Here's how the part is built. I have some questions about the finished solid (model axes, mm). Coordinates: 2 decimals unless noted, no trailing zeros. Loops run counter-clockwise (first coordinate to the right, second up) from the corner with the lowest first, then second, coordinate; pieces in that order, holes last. Notation, with made-up numbers: (63, -15.75) - (88, -15.75) arc R19 ccw to (88, 2.25) - close; hole circle Ø3 at (57.25, 16). An arc over 180 degrees is marked (long way). Use a Markdown table: item, result.
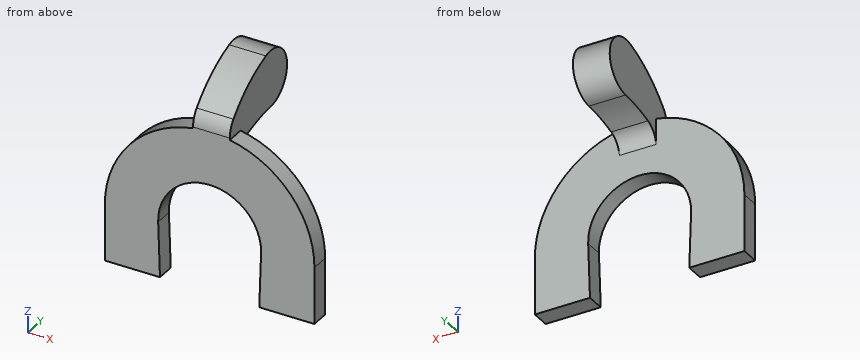
```python
from build123d import *

# Parameters (mm, degrees)
BOSS_EXTRUDE1_DEPTH      = 1
BOSS_EXTRUDE2_START      = 2.8
BOSS_EXTRUDE2_DEPTH      = 1
BOSS_EXTRUDE2_DEPTH_BACK = 1


with BuildPart() as part:
    # Sketch1 → Boss-Extrude1 (new body)
    with BuildSketch(Plane(origin=(0, 0, 0), x_dir=(1, 0, 0), z_dir=(0, 1, 0))):
        with BuildLine():
            Line((0, 0), (-3, 0))
            Line((-3, 0), (-3, -3.090307428))
            ThreePointArc((-3, -3.090307428), (2.7, -8.790307428), (8.4, -3.090307428))
            Line((8.4, -3.090307428), (8.4, 0))
            Line((8.4, 0), (5.4, 0))
            Line((5.4, 0), (5.498490641, -2.99838283))
            ThreePointArc((5.498490641, -2.99838283), (2.7, -5.890307428), (-0.098490641, -2.99838283))
            Line((-0.098490641, -2.99838283), (0, 0))
        make_face()
    extrude(amount=BOSS_EXTRUDE1_DEPTH)

    # Sketch2 → Boss-Extrude2 (add, two sides)
    with BuildSketch(Plane(origin=(0, 0, 0), x_dir=(0, 0, -1), z_dir=(1, 0, 0)).offset(BOSS_EXTRUDE2_START)) as boss_extrude2_sk:
        with BuildLine():
            Line((-6.335210042, 0), (-8.790307428, 0))
            ThreePointArc((-8.790307428, 0), (-9.254427116, 0.08633492), (-9.656455715, 0.333789578))
            ThreePointArc((-9.656455715, 0.333789578), (-10.811745574, 1.711404626), (-11.550251819, 3.350650307))
            ThreePointArc((-11.550251819, 3.350650307), (-10.32088682, 5.296716398), (-8.547723139, 3.828928236))
            ThreePointArc((-8.547723139, 3.828928236), (-8.447124365, 2.781446668), (-8.209910935, 1.756230818))
            ThreePointArc((-8.209910935, 1.756230818), (-7.874898379, 1.24587868), (-7.316117214, 1))
            Line((-7.316117214, 1), (-6.335210042, 1))
            Line((-6.335210042, 1), (-6.335210042, 0))
        make_face()
    extrude(amount=BOSS_EXTRUDE2_DEPTH)
    extrude(boss_extrude2_sk.sketch, amount=-BOSS_EXTRUDE2_DEPTH_BACK)


solid = part.part
```
Q1. Will these pins go through, and if not, where does the flat tip stop? P1, Ø1, axis at y = 2, z = 5.5, coming from the +X side; P2, Ø3, axis at x = 3.5, y = 3, coming from the -Z side; P3, Ø2.5, axis at x = 5, z = 4.5, coming from the +Y side; P4, Ø1.3, axis at y = 2, z = 10.5, coming from the -X side.
Check values:
| item | result |
|---|---|
| P1 | through |
| P2 | z = 8.09 |
| P3 | y = 1 |
| P4 | x = 1.8 |
Q2. I want a section at D-D, the plane x = 4.25. Write out the boundary of the cut face in (y, z).
Check values:
| item | result |
|---|---|
| outline | (0, 5.42) - (1, 5.42) - (1, 8.58) - (0, 8.58) - close |
Q3. I want a section at C-C, the plane y = 2.95. Write out the boundary of the cut face in (x, z).
Check values:
| item | result |
|---|---|
| outline | (1.8, 8.47) - (3.8, 8.47) - (3.8, 11.42) - (1.8, 11.42) - close |
Q4. I want a section at A-A, the plane x = 2.7. Write out the boundary of the cut face in (y, z).
Check values:
| item | result |
|---|---|
| outline | (0, 5.89) - (1, 5.89) - (1, 7.32) arc R1.08 cw to (1.76, 8.21) arc R8 cw to (3.83, 8.55) arc R1.53 ccw (long way) to (3.35, 11.55) arc R6.57 ccw to (0.33, 9.66) arc R1.29 ccw to (0, 8.79) - close |
Q5. I want a section at B-B, the plane z = 4.5. Write out the boundary of the cut face in (x, y), then the cut area to 3 significant figures.
Check values:
| item | result |
|---|---|
| outline | (-2.82, 0) - (0.28, 0) - (0.28, 1) - (-2.82, 1) - close; (5.12, 0) - (8.22, 0) - (8.22, 1) - (5.12, 1) - close |
| area | 6.21 mm^2 |
Q6. Please list where these lines run through material, in increasing order: L1, parallel to Y at x = 6.75, z = 1.75; L2, parallel to X at y = 2.85, z = 9.5; L3, parallel to X at y = 0.6, z = 4.25. Write a range as from..to.
Check values:
| item | result |
|---|---|
| L1 | 0..1 |
| L2 | 1.8..3.8 |
| L3 | -2.88..0.15, 5.25..8.28 |
